Can you work these out from the model? Positions are in its coordinate system, mm. Give positions to 0.01 mm unless a question says otherwise; leave off trailing zeros. Loops run counter-clockwise (first coordinate to the right, second up) from the corner with the lowest first, then second, coordinate; pieces in that order, holes last. Notation, with made-up numbers: (29.5, 36) - (45.5, 36) arc R25 cw to (45.5, 57) - close; hole circle Ø7 at (35, 63). An arc over 180 degrees is marked (long way). Use a Markdown table: item, result. Add a question column.
```python
from build123d import *


with BuildPart() as part:
    # Sketch → Revolution (revolve)
    with BuildSketch(Plane.XZ):
        with BuildLine():
            ThreePointArc((14.075183, -2.166475), (15, 0), (14.075183, 2.166475))
            Line((14.075183, 2.166475), (11.9, 4.25))
            Line((11.9, 4.25), (9.9, 4.25))
            Line((9.9, 4.25), (10.9, 3.25))
            Line((10.9, 0), (10.9, 3.25))
            Line((10.9, 0), (10.9, -3.25))
            Line((10.9, -3.25), (9.9, -4.25))
            Line((11.9, -4.25), (9.9, -4.25))
            Line((14.075183, -2.166475), (11.9, -4.25))
        make_face()
    revolve(axis=Axis((0, 0, 0), (0, 0, 1)))


solid = part.part
```
1. Suppose I cut it at D-D (z = 2.75). List the corners of the cut face in (x, y) for me.
2. Suppose I cut it at A-A (y = 0). List the corners of the cut face in (x, z) for me.
3. Suppose I cut it at C-C (z = -1.75). List the corners of the cut face in (x, y) for me.
4. Will these pins go through, and if not, where does the flat tip stop? P1, Ø17.5, axis at x = 0, y = 0, coming from the -Z side; P2, Ø2, axis at y = 9, z = 1, coming from the -X side; P3, Ø3, axis at y = 7, z = 2.5, coming from the +X side.
5. Please list where these lines run through material, in increasing order: line 1 along X through (y, z) = (-1, -2.75); line 2 along Y through (x, z) = (0, -1.25); line 3 along X through (y, z) = (1, -0.5). Write a range as [from, to].
6. If we mould it in two halves opening along X, with no side actions, what happens to faces 1 (the face through (-10, 2, -4.25)), 2 (the face through (10.4, 3.27, -0.05))? For each: released by +X, released by -X, zero draft, split by the parting line, or undercut.
Results below:
| question | item | result |
|---|---|---|
| 1 | outline | circle Ø26.93 at (0, 0); hole circle Ø21.8 at (0, 0) |
| 2 | outline | (-14.08, -2.17) - (-11.9, -4.25) - (-9.9, -4.25) - (-10.9, -3.25) - (-10.9, 3.25) - (-9.9, 4.25) - (-11.9, 4.25) - (-14.08, 2.17) arc R3 ccw to start; (9.9, -4.25) - (11.9, -4.25) - (14.08, -2.17) arc R3 ccw to (14.08, 2.17) - (11.9, 4.25) - (9.9, 4.25) - (10.9, 3.25) - (10.9, -3.25) - close |
| 3 | outline | circle Ø28.87 at (0, 0); hole circle Ø21.8 at (0, 0) |
| 4 | P1 | through |
| 4 | P2 | x = -12.56 |
| 4 | P3 | x = 13.38 |
| 5 | line 1 | [-13.43, -10.85], [10.85, 13.43] |
| 5 | line 2 | [-14.73, -10.9], [10.9, 14.73] |
| 5 | line 3 | [-14.92, -10.85], [10.85, 14.92] |
| 6 | face 1 | zero draft |
| 6 | face 2 | undercut |
